The listing builds one solid part. Answer for the finished solid, in the listing's coordinates (mm). Face numbers are marked on the shaded views. A direction names the side the tool comes from. Coordinates: 2 decimals unless noted, no trailing zeros. Write each loop counter-clockwise with the first axis right and the second up, starting at its lowest first coordinate (ties: lowest second). Pieces come first, ordered by that corner, then holes. Notation, with made-up numbers: M 66.25,-21.75 L 99.25,-21.75 A25 ccw 99.25,15.25 Z; hole C -31.75,-34.75 d3. An arc over 180 degrees is marked long. Answer as CSV lines item,"result".
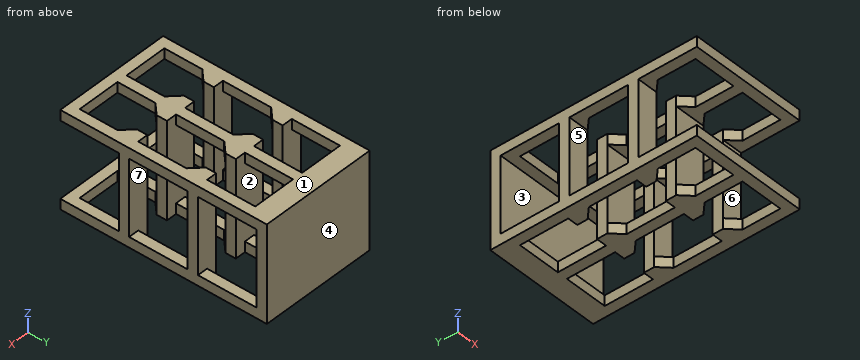
```python
from build123d import *

# Parameters (mm, degrees)
SKETCH1_W               = 340
SKETCH1_H               = 280
BOSS_EXTRUDE1_DEPTH     = 600
CUT_EXTRUDE1_DEPTH      = 704.70448343
CUT_EXTRUDE1_DEPTH_BACK = 704.70448343
SKETCH4_W               = 220
SKETCH4_H               = 170
CUT_EXTRUDE3_DEPTH      = 684.593446429
CUT_EXTRUDE3_DEPTH_BACK = 684.593446429
SKETCH6_W               = 125
SKETCH6_H               = 110


with BuildPart() as part:
    # Sketch1 → Boss-Extrude1 (new body)
    with BuildSketch(Plane(origin=(0, 0, 0), x_dir=(1, 0, 0), z_dir=(0, 1, 0))):
        Rectangle(SKETCH1_W, SKETCH1_H)
    extrude(amount=BOSS_EXTRUDE1_DEPTH)

    # Sketch4 → Cut-Extrude1 (cut, two sides: drawn at the far end of the back side and taken through both)
    with BuildSketch(Plane(origin=(170, 0, 0), x_dir=(0, 0, -1), z_dir=(1, 0, 0)).offset(-CUT_EXTRUDE1_DEPTH_BACK)):
        with Locations((0, 485)):
            Rectangle(SKETCH4_W, SKETCH4_H)
        with Locations((0, 285)):
            Rectangle(SKETCH4_W, SKETCH4_H)
        with Locations((0, 85)):
            Rectangle(SKETCH4_W, SKETCH4_H)
    extrude(amount=CUT_EXTRUDE1_DEPTH + CUT_EXTRUDE1_DEPTH_BACK, mode=Mode.SUBTRACT)

    # Sketch6 → Cut-Extrude3 (cut, two sides: drawn at the far end of the back side and taken through both)
    with BuildSketch(Plane.XY.offset(140).offset(-CUT_EXTRUDE3_DEPTH_BACK)):
        Polygon((-15, 540), (-140, 540), (-140, 400), (-110, 400), (-110, 370), (-45, 370), (-45, 400), (-15, 400), align=None)
        Polygon((140, 540), (15, 540), (15, 400), (45, 400), (45, 370), (110, 370), (110, 400), (140, 400), align=None)
        Polygon((140, 340), (15, 340), (15, 200), (45, 200), (45, 170), (110, 170), (110, 200), (140, 200), align=None)
        Polygon((-15, 340), (-140, 340), (-140, 200), (-110, 200), (-110, 170), (-45, 170), (-45, 200), (-15, 200), align=None)
        with Locations((-77.5, 85)):
            Rectangle(SKETCH6_W, SKETCH6_H)
        with Locations((77.5, 85)):
            Rectangle(SKETCH6_W, SKETCH6_H)
        Polygon((-45, 170), (-110, 170), (-140, 140), (-15, 140), align=None)
        Polygon((110, 170), (45, 170), (15, 140), (140, 140), align=None)
        Polygon((110, 370), (45, 370), (15, 340), (140, 340), align=None)
        Polygon((-45, 370), (-110, 370), (-140, 340), (-15, 340), align=None)
    extrude(amount=CUT_EXTRUDE3_DEPTH + CUT_EXTRUDE3_DEPTH_BACK, mode=Mode.SUBTRACT)


solid = part.part
```
Q1. The mould has two halves that part along Y. Classify the marked faces 1, 2, 3 and 4: pulls with the +Y half, pulls with the -Y half, needs draft (parallel to the pull), parting line crosses it, or undercut.
Output:
face 1,"needs draft"
face 2,"undercut"
face 3,"undercut"
face 4,"pulls with the +Y half"
Q2. Straight lines are drawn through the part: line 1 (Y direction, x = -29.5, z = -107); line 2 (X direction, y = 173, z = -122.5); line 3 (X direction, y = 34.5, z = -123). For each, find the intervals that lie inside material, in ascending order.
Output:
line 1,"170 to 200, 370 to 400, 570 to 600"
line 2,"-170 to -110, -45 to 45, 110 to 170"
line 3,"-170 to -140, -15 to 15, 140 to 170"
Q3. Find section A-A (y = 310). Give the vertices of the cut face in (x, z), and give its area (3 significant figures).
Output:
outline,"M -170,-140 L -140,-140 L -140,-110 L -170,-110 Z; M -170,110 L -140,110 L -140,140 L -170,140 Z; M -15,-140 L 15,-140 L 15,-110 L -15,-110 Z; M -15,110 L 15,110 L 15,140 L -15,140 Z; M 140,-140 L 170,-140 L 170,-110 L 140,-110 Z; M 140,110 L 170,110 L 170,140 L 140,140 Z"
area,"5,400 mm2"
Q4. For the marked faces 5, 6 and 7, determine the directions among +Z, -Z, +X, -X, +Y, -Y from which every point of the face is accessible in a straight line to the end or side of a thin tool.
Output:
face 5,"+X, -X"
face 6,"+X, -X, -Y"
face 7,"none"
Q5. Flat-ended cylindrical pins translate along their axes: pin 1 Ø15 at (x, z) = (-53, 127.5) entering from -Y; pin 2 Ø10 at (x, z) = (-117, 70.5) entering from -Y. Find the tip coordinate at first contact, or state that the pin passes through.
Output:
pin 1,"y = 0"
pin 2,"y = 170"
Q6. Find section B-B (z = 48). Give the vertices of the cut face in (x, y).
Output:
outline,"M -170,170 L -110,170 L -110,200 L -170,200 Z; M -170,370 L -110,370 L -110,400 L -170,400 Z; M -170,570 L 170,570 L 170,600 L -170,600 Z; M -45,170 L 45,170 L 45,200 L -45,200 Z; M -45,370 L 45,370 L 45,400 L -45,400 Z; M 110,170 L 170,170 L 170,200 L 110,200 Z; M 110,370 L 170,370 L 170,400 L 110,400 Z"
Q7. Find section C-C (x = -62). Give the vertices of the cut face in (y, z), and give its area (3 significant figures).
Output:
outline,"M 0,-140 L 30,-140 L 30,-110 L 0,-110 Z; M 0,110 L 30,110 L 30,140 L 0,140 Z; M 540,-140 L 600,-140 L 600,140 L 540,140 L 540,110 L 570,110 L 570,-110 L 540,-110 Z"
area,"12,000 mm2"
Q8. Find section D-D (y = 546). Give the vertices of the cut face in (x, z).
Output:
outline,"M -170,-140 L 170,-140 L 170,-110 L -170,-110 Z; M -170,110 L 170,110 L 170,140 L -170,140 Z"
